from build123d import *

# Parameters (mm, degrees)
BOSS_EXTRUDE1_DEPTH                                 = 5
CBORE_FOR_4_BINDING_HEAD_MACHINE_SCREW1_D           = 3.2639
CBORE_FOR_4_BINDING_HEAD_MACHINE_SCREW1_DEPTH       = 5
CBORE_FOR_4_BINDING_HEAD_MACHINE_SCREW1_CBORE_D     = 6.74624
CBORE_FOR_4_BINDING_HEAD_MACHINE_SCREW1_CBORE_DEPTH = 1.7272


with BuildPart() as part:
    # Sketch1 → Boss-Extrude1 (new body)
    with BuildSketch(Plane(origin=(0, 0, 0), x_dir=(1, 0, 0), z_dir=(0, 1, 0))):
        with BuildLine():
            Line((109.044117647, 56.029411765), (-70.955882353, 56.029411765))
            Line((-70.955882353, 56.029411765), (-70.955882353, -18.970588235))
            Line((-70.955882353, -18.970588235), (-15.955882353, -18.970588235))
            ThreePointArc((-15.955882353, -18.970588235), (-12.420348447, -20.435054329), (-10.955882353, -23.970588235))
            Line((-10.955882353, -23.970588235), (-10.955882353, -93.970588235))
            Line((-10.955882353, -93.970588235), (109.044117647, -93.970588235))
            Line((109.044117647, -93.970588235), (109.044117647, -18.970588235))
            Line((109.044117647, -18.970588235), (109.044117647, 56.029411765))
        make_face()
    extrude(amount=BOSS_EXTRUDE1_DEPTH)

    # CBORE for #4 Binding Head Machine Screw1
    with Locations(Plane(origin=(0, 5, 0), x_dir=(1, 0, 0), z_dir=(0, 1, 0))):
        with Locations((-65.955882353, 51.029411765), (-65.955882353, -11.470588235), (-5.845882353, -11.470588235), (-5.845882353, -88.970588235), (104.044117647, -88.970588235), (104.044117647, 51.029411765)):
            CounterBoreHole(CBORE_FOR_4_BINDING_HEAD_MACHINE_SCREW1_D / 2, CBORE_FOR_4_BINDING_HEAD_MACHINE_SCREW1_CBORE_D / 2, CBORE_FOR_4_BINDING_HEAD_MACHINE_SCREW1_CBORE_DEPTH, depth=CBORE_FOR_4_BINDING_HEAD_MACHINE_SCREW1_DEPTH)


solid = part.part
For this review, take the finished solid that the model builds, in its own axes (mm). A direction names the side the tool comes from. Coordinates: 2 decimals unless noted, no trailing zeros. Loops run counter-clockwise (first coordinate to the right, second up) from the corner with the lowest first, then second, coordinate; pieces in that order, holes last. Notation, with made-up numbers: (3.5, 59.25) - (12.5, 59.25) arc R24 ccw to (12.5, 79.25) - close; hole circle Ø7 at (78.25, 14.25). An arc over 180 degrees is marked (long way). Use a Markdown table: item, result. Add a question column.
Item 1: We need section A-A (y = 1.35). Give the boundary of the cut face in (x, z).
Item 2: We need section B-B (z = 38). Give the boundary of the cut face in (x, y), and give its area (3 significant figures).
Item 3: Tool access review of faces 1 (the face through (38, 5, 18)), 2 (the face through (-6.285, 4.148, 85.626)), 3 (the face through (-10.956, 2, 58)): name each direction out of +Z, -Z, +X, -X, +Y, -Y from which nothing blocks a thin tool from reaching the whole face with its end or side.
Item 4: Insertion check: pin 1 Ø7.5 at (x, z) = (-65.5, -50) entering from +Y; pin 2 Ø2 at (x, z) = (104.04, -51.03) entering from +Y; pin 3 Ø3.5 at (x, z) = (-7, 89) entering from +Y; pin 4 Ø2.5 at (x, y) = (-37.5, 3.5) entering from +Z. Each pin has a flat end and moves straight along its axis. Give the tip position at first contact, or say it passes through.
Item 5: We need section C-C (x = -28). Give the boundary of the cut face in (y, z).
Item 6: Mouldability with a two-part tool opening along X and no side actions: class faces 4 (the face through (105, 3.273, 87)), 5 (the face through (109.044, 2, 20)), 6 (the face through (-44, 2, 18.971)) as pulls with the +X half, pulls with the -X half, needs draft (parallel to the pull), parting line crosses it, or undercut.
Item 7: For line 1 (X direction, y = 2.2, z = 11); line 2 (X direction, y = 2.45, z = 73); line 3 (Z direction, x = -56, y = 3.3), list the stretches that pass through material, from the lowest coordinate up.
Results list:
| question | item | result |
|---|---|---|
| 1 | outline | (-70.96, -56.03) - (109.04, -56.03) - (109.04, 93.97) - (-10.96, 93.97) - (-10.96, 23.97) arc R5 cw to (-15.96, 18.97) - (-70.96, 18.97) - close; hole circle Ø3.26 at (-65.96, -51.03); hole circle Ø3.26 at (-65.96, 11.47); hole circle Ø3.26 at (-5.85, 11.47); hole circle Ø3.26 at (-5.85, 88.97); hole circle Ø3.26 at (104.04, -51.03); hole circle Ø3.26 at (104.04, 88.97) |
| 2 | outline | (-10.96, 0) - (109.04, 0) - (109.04, 5) - (-10.96, 5) - close |
| 2 | area | 600 mm^2 |
| 3 | face 1 | +Z, -Z, +X, -X, +Y |
| 3 | face 2 | +Y |
| 3 | face 3 | +Z, -X, +Y, -Y |
| 4 | pin 1 | stops at y = 5 |
| 4 | pin 2 | passes through |
| 4 | pin 3 | stops at y = 3.27 |
| 4 | pin 4 | stops at z = 18.97 |
| 5 | outline | (0, -56.03) - (5, -56.03) - (5, 18.97) - (0, 18.97) - close |
| 6 | face 4 | undercut |
| 6 | face 5 | pulls with the +X half |
| 6 | face 6 | needs draft |
| 7 | line 1 | x = -70.96 to -67.52, -64.39 to -7.41, -4.28 to 109.04 |
| 7 | line 2 | x = -10.96 to 109.04 |
| 7 | line 3 | z = -56.03 to 18.97 |
